```python
from build123d import *

# Parameters (mm, degrees)
SKETCH_1_R          = 1.6
SKETCH_1_R_2        = 0.64
EXTRUDE_1_DEPTH     = 50
SKETCH_4_W          = 155.949110162
SKETCH_4_H          = 42
CUT_EXTRUDE_3_DEPTH = 21
SKETCH_5_W          = 23
SKETCH_5_H          = 9.401567806
SKETCH_5_W_2        = 49
CUT_EXTRUDE_4_DEPTH = 51
SKETCH_6_W          = 4.324691993
SKETCH_6_H          = 28
CUT_EXTRUDE_5_DEPTH = 215.974555081
SKETCH_7_W          = 143.949110162
SKETCH_7_H          = 2
CUT_EXTRUDE_6_DEPTH = 21


with BuildPart() as part:
    # 草图1 → 凸台-拉伸1 (new body)
    with BuildSketch(Plane(origin=(0, 0, 0), x_dir=(1, 0, 0), z_dir=(0, 1, 0))):
        with BuildLine():
            Line((-163.25203252, 10), (76.74796748, 10))
            ThreePointArc((76.74796748, 10), (86.74796748, 0), (76.74796748, -10))
            Line((76.74796748, -10), (-163.25203252, -10))
            ThreePointArc((-163.25203252, -10), (-173.25203252, 0), (-163.25203252, 10))
        make_face()
        with Locations((76.74796748, 0)):
            Circle(SKETCH_1_R, mode=Mode.SUBTRACT)
        with Locations((-163.25203252, 0)):
            Circle(SKETCH_1_R, mode=Mode.SUBTRACT)
        with Locations((-59.25203252, 0)):
            Circle(SKETCH_1_R_2, mode=Mode.SUBTRACT)
        with Locations((-43.25203252, 0)):
            Circle(SKETCH_1_R, mode=Mode.SUBTRACT)
        with Locations((-27.25203252, 0)):
            Circle(SKETCH_1_R_2, mode=Mode.SUBTRACT)
    extrude(amount=EXTRUDE_1_DEPTH)

    # 草图4 → 切除-拉伸3 (cut, through all)
    with BuildSketch(Plane(origin=(0, 0, -10), x_dir=(-1, 0, 0), z_dir=(0, 0, -1))):
        Polygon((-86.722522561, 45), (-56.74796748, 45), (-41.722522561, 45), (-41.722522561, 5), (-56.74796748, 5), (-86.74796748, 5), (-94.689865515, 5), (-94.689865515, 45), align=None)
        Polygon((128.226587601, 5), (173.25203252, 5), (178.626350661, 5), (178.626350661, 45), (173.226587601, 45), (128.226587601, 45), align=None)
        with Locations((43.25203252, 21)):
            Rectangle(SKETCH_4_W, SKETCH_4_H)
    extrude(amount=-CUT_EXTRUDE_3_DEPTH, mode=Mode.SUBTRACT)

    # 草图5 → 切除-拉伸4 (cut, through all)
    with BuildSketch(Plane.XZ):
        with Locations((58.222522561, 0)):
            Rectangle(SKETCH_5_W, SKETCH_5_H)
        with Locations((4.222522561, 0)):
            Rectangle(SKETCH_5_W_2, SKETCH_5_H)
        with Locations((-90.726587601, 0)):
            Rectangle(SKETCH_5_W_2, SKETCH_5_H)
        with Locations((-144.726587601, 0)):
            Rectangle(SKETCH_5_W, SKETCH_5_H)
    extrude(amount=-CUT_EXTRUDE_4_DEPTH, mode=Mode.SUBTRACT)

    # 草图6 → 切除-拉伸5 (cut, through all)
    with BuildSketch(Plane.ZY.offset(128.226587601)):
        with Locations((1.837654003, 25)):
            Rectangle(SKETCH_6_W, SKETCH_6_H)
    extrude(amount=-CUT_EXTRUDE_5_DEPTH, mode=Mode.SUBTRACT)

    # 草图7 → 切除-拉伸6 (cut, through all)
    with BuildSketch(Plane.XY.offset(10)):
        with Locations((-43.25203252, 49)):
            Rectangle(SKETCH_7_W, SKETCH_7_H)
    extrude(amount=-CUT_EXTRUDE_6_DEPTH, mode=Mode.SUBTRACT)


solid = part.part
```
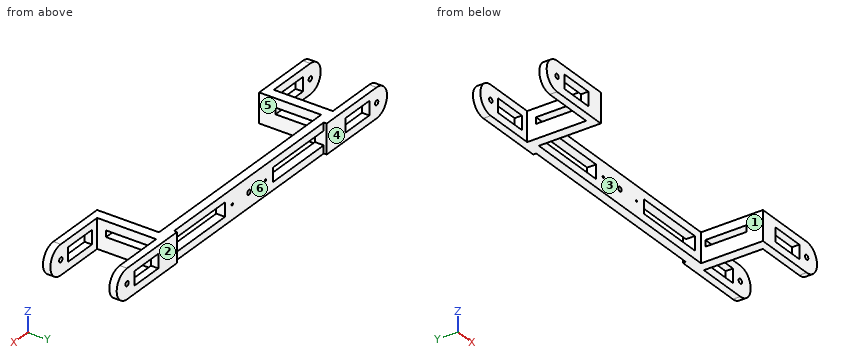
For this review, take the finished solid that the model builds, in its own axes (mm). Face numbers are marked on the shaded views. A direction names the side the tool comes from. Coordinates: 2 decimals unless noted, no trailing zeros. Loops run counter-clockwise (first coordinate to the right, second up) from the corner with the lowest first, then second, coordinate; pieces in that order, holes last.
1. Add section A-A, the plane y = 14.5. Give the boundary of the cut face in (x, z), then the cut area to 3 significant figures.
2. Add section B-B, the plane x = -7. Give the boundary of the cut face in (y, z), then the cut area to 3 significant figures.
3. Add section C-C, the plane x = -53.5. Give the boundary of the cut face in (y, z).
4. Insertion check: P1, Ø4, axis at y = 43.5, z = 3.5, coming from the +X side; P2, Ø6, axis at x = -62.5, z = 4.5, coming from the -Y side; P3, Ø2.5, axis at y = 3.5, z = -1.5, coming from the +X side; P4, Ø2, axis at y = 15.5, z = 2, coming from the -X side. Each pin has a flat end and moves straight along its axis. Give the tip position at first contact, or say it passes through.
5. Mouldability with a two-part tool opening along X and no side actions: class the marked faces 1, 2 and 3 as +X half, -X half, draft (parallel to the pull), parting line (faces both ways), or undercut.
6. For the marked faces 4, 5 and 6, list the 3-axis set-ups (+Z, -Z, +X, -X, +Y, -Y) from which the entire face can be reached by the end or side of a thin tool; tool diameter is ignored.
7. For line 1 (X direction, y = 3.15, z = 0); line 2 (X direction, y = 8, z = -8.75); line 3 (X direction, y = 4, z = -1), list the stretches that pass through material, from the lowest coordinate up.
Result:
1. outline: (-128.23, -10) - (-121.23, -10) - (-121.23, -0.32) - (-128.23, -0.32) - close; (-128.23, 4) - (-121.23, 4) - (-121.23, 10) - (-128.23, 10) - close; (34.72, -10) - (41.72, -10) - (41.72, -0.32) - (34.72, -0.32) - close; (34.72, 4) - (41.72, 4) - (41.72, 10) - (34.72, 10) - close
1. area: 219 mm2
2. outline: (42, -10) - (48, -10) - (48, -4.7) - (42, -4.7) - close; (42, 4.7) - (48, 4.7) - (48, 10) - (42, 10) - close
2. area: 63.6 mm2
3. outline: (42, -10) - (48, -10) - (48, 10) - (42, 10) - close
4. P1: stops at x = 86.51
4. P2: stops at y = 42
4. P3: stops at x = 86.74
4. P4: passes through
5. face 1: undercut
5. face 2: draft
5. face 3: undercut
6. face 4: +Z, -Z, +X, -X, +Y
6. face 5: +Z, -Z, -Y
6. face 6: +Z, -Z, +Y
7. line 1: x = -173.25 to -164.85, -161.65 to -156.23, -133.23 to -121.23, 34.72 to 46.72, 69.72 to 75.15, 78.35 to 86.75
7. line 2: x = -128.23 to -121.23, 34.72 to 41.72
7. line 3: x = -173.2 to -164.5, -162 to -156.23, -133.23 to -121.23, 34.72 to 46.72, 69.72 to 75.5, 78 to 86.7
